Check sheet for the modelled part. Datum: model origin and axes. Units: mm. A direction names the side the tool comes from. Round coordinates to 2 decimals unless told otherwise and drop trailing zeros. Order: outer loops, then holes, each group sorted by start corner. A loop starts at its lowest first (then second) coordinate and runs counter-clockwise, first axis right, second up.
(1) Sectioned sample at A-A, the plane x = 0. Enter the section's corners in (y, z), and give its area (3 significant figures).
(2) Sectioned sample at B-B, the plane z = -4.25. Enter the section's corners in (x, y) (3 decimals), and give its area (3 significant figures).
(3) Tool access check on faces 4 (the cylindrical face through (-21.977, 18.252, -3.01)), 5 (the flat face through (-25.445, 0, -6)), 6 (the flat face through (-22, -13.5, -4)). Record the directions out of +Z, -Z, +X, -X, +Y, -Y that give a thin tool (end or side, any length) a straight path to the whole face; none if there is none.
(4) Depth check by flat-ended pin: pin 1 (1.8 mm diameter, centred on y = -20.5, z = -4.5, fed in from +X); pin 2 (1.1 mm diameter, centred on y = -23.5, z = -11.5, fed in from -X); pin 3 (1.8 mm diameter, centred on y = -21.5, z = -6, fed in from -X); pin 4 (10 mm diameter, centred on x = -20, y = -16.5, fed in from -Z). Enter the tip coordinate at first touch or a pass-through.
(5) Sectioned sample at D-D, the plane y = -10.5. Enter the section's corners in (x, z) (3 decimals).
(6) Thickness scan on probe 1 along Y at (x, z) = (-18.98, -7.9); probe 2 along X at (y, z) = (14.5, -11) (3 decimals); probe 3 along Y at (x, z) = (-4.5, -5). Record the ranges inside material, lowest first.
(7) Sectioned sample at C-C, the plane y = -2.5. Enter the section's corners in (x, z) (3 decimals), and give its area (3 significant figures).
(8) Mould release check, pull along X, two halves, no side actions. Record for faces 1 (the flat face through (24.445, 0, -7)), 2 (the conical face through (-23.062, -21.933, 0.64)), 3 (the cylindrical face through (23.566, 22.618, -6.313)): released by +X, released by -X, zero draft, split by the parting line, or undercut.
```python
from build123d import *

# Parameters (mm, degrees)
SKETCH_R        = 6.1
PAD_DEPTH       = 0.8
PAD001_DEPTH    = 12.6
CHAMFER_SIZE    = 1
PAD002_DEPTH    = 8.4
SKETCH003_W     = 5.4
SKETCH003_H     = 2.7
POCKET_DEPTH    = 2
CHAMFER001_SIZE = 1


with BuildPart() as part:
    # Sketch → Pad (new body)
    with BuildSketch(Plane.XY):
        with BuildLine():
            Line((-19.195, 24.4), (19.195, 24.4))
            ThreePointArc((25.445, 18.15), (23.614417, 22.569417), (19.195, 24.4))
            Line((25.445, 18.15), (25.445, -18.15))
            ThreePointArc((19.195, -24.4), (23.614417, -22.569417), (25.445, -18.15))
            Line((19.195, -24.4), (-19.195, -24.4))
            ThreePointArc((-25.445, -18.15), (-23.614417, -22.569417), (-19.195, -24.4))
            Line((-25.445, -18.15), (-25.445, 18.15))
            ThreePointArc((-19.195, 24.4), (-23.614417, 22.569417), (-25.445, 18.15))
        make_face()
        with Locations((-15.25, 0)):
            Circle(SKETCH_R, mode=Mode.SUBTRACT)
        Circle(SKETCH_R, mode=Mode.SUBTRACT)
        with Locations((15.25, 0)):
            Circle(SKETCH_R, mode=Mode.SUBTRACT)
        with Locations((0, 15.25)):
            Circle(SKETCH_R, mode=Mode.SUBTRACT)
        with Locations((0, -15.25)):
            Circle(SKETCH_R, mode=Mode.SUBTRACT)
    extrude(amount=PAD_DEPTH)

    # Sketch005 (on Face14 of Pad) → Pad001 (join)
    with BuildSketch(Plane(origin=(0, 0, 0), x_dir=(1, 0, 0), z_dir=(0, 0, -1))):
        with BuildLine():
            Line((-19.195, 24.4), (19.195, 24.4))
            ThreePointArc((25.445, 18.15), (23.614417, 22.569417), (19.195, 24.4))
            Line((25.445, 18.15), (25.445, -18.15))
            ThreePointArc((19.195, -24.4), (23.614417, -22.569417), (25.445, -18.15))
            Line((19.195, -24.4), (-19.195, -24.4))
            ThreePointArc((-25.445, -18.15), (-23.614417, -22.569417), (-19.195, -24.4))
            Line((-25.445, -18.15), (-25.445, 18.15))
            ThreePointArc((-19.195, 24.4), (-23.614417, 22.569417), (-25.445, 18.15))
        make_face()
        with BuildLine():
            Line((-19.195, 23.4), (19.195, 23.4))
            ThreePointArc((24.445, 18.15), (22.907311, 21.862311), (19.195, 23.4))
            Line((24.445, 18.15), (24.445, -18.15))
            ThreePointArc((19.195, -23.4), (22.907311, -21.862311), (24.445, -18.15))
            Line((19.195, -23.4), (-19.195, -23.4))
            ThreePointArc((-24.445, -18.15), (-22.907311, -21.862311), (-19.195, -23.4))
            Line((-24.445, -18.15), (-24.445, 18.15))
            ThreePointArc((-19.195, 23.4), (-22.907311, 21.862311), (-24.445, 18.15))
        make_face(mode=Mode.SUBTRACT)
    extrude(amount=PAD001_DEPTH)

    # Chamfer
    chamfer_edges = [part.edges().sort_by_distance(p)[0] for p in [
        (-22.907311, 21.862311, 0),
        (23.614417, 22.569417, 0.8),
    ]]
    chamfer(chamfer_edges, length=CHAMFER_SIZE)

    # Sketch006 → Pad002 (join)
    with BuildSketch(Plane.XY):
        with BuildLine():
            ThreePointArc((-19.195, 23.4), (-22.907311, 21.862311), (-24.445, 18.15))
            Line((-24.445, 18.15), (-24.445, 14.12))
            Line((-19.14, 14.12), (-24.445, 14.12))
            ThreePointArc((-19.14, 14.12), (-16.311573, 15.291573), (-15.14, 18.12))
            Line((-15.14, 18.12), (-15.14, 23.4))
            Line((-19.195, 23.4), (-15.14, 23.4))
        make_face()
        with BuildLine():
            ThreePointArc((24.445, 18.15), (22.907311, 21.862311), (19.195, 23.4))
            Line((14.96, 23.4), (19.195, 23.4))
            Line((14.96, 18.12), (14.96, 23.4))
            ThreePointArc((14.96, 18.12), (16.131573, 15.291573), (18.96, 14.12))
            Line((18.96, 14.12), (24.445, 14.12))
            Line((24.445, 18.15), (24.445, 14.12))
        make_face()
        with BuildLine():
            ThreePointArc((19.195, -23.4), (22.907311, -21.862311), (24.445, -18.15))
            Line((24.445, -13.5), (24.445, -18.15))
            Line((18.96, -13.5), (24.445, -13.5))
            ThreePointArc((18.96, -13.5), (16.131573, -14.671573), (14.96, -17.5))
            Line((14.96, -17.5), (14.96, -23.4))
            Line((14.96, -23.4), (19.195, -23.4))
        make_face()
        with BuildLine():
            ThreePointArc((-24.445, -18.15), (-22.907311, -21.862311), (-19.195, -23.4))
            Line((-19.195, -23.4), (-15.14, -23.4))
            Line((-15.14, -17.5), (-15.14, -23.4))
            ThreePointArc((-15.14, -17.5), (-16.311573, -14.671573), (-19.14, -13.5))
            Line((-19.14, -13.5), (-24.445, -13.5))
            Line((-24.445, -13.5), (-24.445, -18.15))
        make_face()
    extrude(amount=-PAD002_DEPTH)

    # Sketch004 → Groove (revolve, cut)
    with BuildSketch(Plane(origin=(-18.98, 18.12, 0), x_dir=(1, 0, 0), z_dir=(0, -1, 0))):
        Polygon((3, 2), (0, 2), (0, -11), (1.6, -11), (1.6, -7.3), (3, -5.9), align=None)
    revolve(axis=Axis((-18.98, 18.12, 0), (0, 0, 1)), mode=Mode.SUBTRACT)

    # Sketch007 → Groove001 (revolve, cut)
    with BuildSketch(Plane(origin=(19.12, -17.5, 0), x_dir=(1, 0, 0), z_dir=(0, -1, 0))):
        Polygon((0, -11), (1.6, -11), (1.6, -7.3), (3, -5.9), (3, 2), (0, 2), align=None)
    revolve(axis=Axis((19.12, -17.5, 0), (0, 0, 1)), mode=Mode.SUBTRACT)

    # Sketch003 (on Face16 of Groove001) → Pocket (cut)
    with BuildSketch(Plane.XZ.offset(24.4)):
        with Locations((-12, -11.35)):
            Rectangle(SKETCH003_W, SKETCH003_H)
    extrude(amount=-POCKET_DEPTH, mode=Mode.SUBTRACT)

    # Chamfer001
    chamfer001_edges = [part.edges().sort_by_distance(p)[0] for p in [
        (16.12, -17.5, 0.8),
        (-21.98, 18.12, 0.8),
    ]]
    chamfer(chamfer001_edges, length=CHAMFER001_SIZE)


solid = part.part
```
Derived:
1. outline: (-24.4, -12.6) - (-23.4, -12.6) - (-23.4, -1) - (-22.4, 0) - (-21.35, 0) - (-21.35, 0.8) - (-23.4, 0.8) - (-24.4, -0.2) - close; (-9.15, 0) - (-6.1, 0) - (-6.1, 0.8) - (-9.15, 0.8) - close; (6.1, 0) - (9.15, 0) - (9.15, 0.8) - (6.1, 0.8) - close; (21.35, 0) - (22.4, 0) - (23.4, -1) - (23.4, -12.6) - (24.4, -12.6) - (24.4, -0.2) - (23.4, 0.8) - (21.35, 0.8) - close
1. area: 35.0 mm2
2. outline: (-25.445, -18.15) arc R6.25 ccw to (-19.195, -24.4) - (19.195, -24.4) arc R6.25 ccw to (25.445, -18.15) - (25.445, 18.15) arc R6.25 ccw to (19.195, 24.4) - (-19.195, 24.4) arc R6.25 ccw to (-25.445, 18.15) - close; hole (-24.445, -13.5) - (-19.14, -13.5) arc R4 cw to (-15.14, -17.5) - (-15.14, -23.4) - (14.96, -23.4) - (14.96, -17.5) arc R4 cw to (18.96, -13.5) - (24.445, -13.5) - (24.445, 14.12) - (18.96, 14.12) arc R4 cw to (14.96, 18.12) - (14.96, 23.4) - (-15.14, 23.4) - (-15.14, 18.12) arc R4 cw to (-19.14, 14.12) - (-24.445, 14.12) - close; hole circle Ø6 at (-18.98, 18.12); hole circle Ø6 at (19.12, -17.5)
2. area: 452 mm2
3. face 4: +Z
3. face 5: +Z, -Z, -X, +Y, -Y
3. face 6: -Z
4. pin 1: stops at x = 25.27
4. pin 2: stops at x = -23.2
4. pin 3: stops at x = -24.94
4. pin 4: stops at z = -12.6
5. outline: (-25.445, -12.6) - (-24.445, -12.6) - (-24.445, -1) - (-23.445, 0) - (-3.827, 0) - (-3.827, 0.8) - (-24.445, 0.8) - (-25.445, -0.2) - close; (3.827, 0) - (23.445, 0) - (24.445, -1) - (24.445, -12.6) - (25.445, -12.6) - (25.445, -0.2) - (24.445, 0.8) - (3.827, 0.8) - close
6. probe 1: y = -24.4 to -13.5, 14.12 to 16.52, 19.72 to 24.4
6. probe 2: x = -25.445 to -24.445, 24.445 to 25.445
6. probe 3: y = -24.4 to -23.4, 23.4 to 24.4
7. outline: (-25.445, -12.6) - (-24.445, -12.6) - (-24.445, -1) - (-23.445, 0) - (-20.814, 0) - (-20.814, 0.8) - (-24.445, 0.8) - (-25.445, -0.2) - close; (-9.686, 0) - (-5.564, 0) - (-5.564, 0.8) - (-9.686, 0.8) - close; (5.564, 0) - (9.686, 0) - (9.686, 0.8) - (5.564, 0.8) - close; (20.814, 0) - (23.445, 0) - (24.445, -1) - (24.445, -12.6) - (25.445, -12.6) - (25.445, -0.2) - (24.445, 0.8) - (20.814, 0.8) - close
7. area: 39.2 mm2
8. face 1: undercut
8. face 2: released by -X
8. face 3: released by +X
